from build123d import *

# Parameters (mm, degrees)
IZIM1_W                     = 40
IZIM1_H                     = 48
Y_KSEKLIK_EKSTR_ZYON1_DEPTH = 16
RADYUS4_R                   = 4
IZIM5_W                     = 24
IZIM5_H                     = 8
KES_EKSTR_ZYON1_DEPTH       = 59
IZIM6_W                     = 55
IZIM6_H                     = 32
Y_KSEKLIK_EKSTR_ZYON4_DEPTH = 12
RADYUS7_R                   = 10
IZIM9_R                     = 4.2
KES_EKSTR_ZYON2_DEPTH       = 21
IZIM10_W                    = 7
IZIM10_H                    = 35
Y_KSEKLIK_EKSTR_ZYON5_DEPTH = 16
KES_EKSTR_ZYON3_DEPTH       = 16


with BuildPart() as part:
    # Çizim1 → Yükseklik-Ekstrüzyon1 (new body)
    with BuildSketch(Plane.XY):
        with Locations((-20, 24)):
            Rectangle(IZIM1_W, IZIM1_H)
    extrude(amount=Y_KSEKLIK_EKSTR_ZYON1_DEPTH)

    # Radyus4
    radyus4_edges = [part.edges().sort_by_distance(p)[0] for p in [
        (-40, 24, 16),
        (0, 24, 16),
    ]]
    fillet(radyus4_edges, radius=RADYUS4_R)

    # Çizim5 → Kes-Ekstrüzyon1 (cut)
    with BuildSketch(Plane(origin=(0, 48, 0), x_dir=(1, 0, 0), z_dir=(0, 1, 0))):
        with Locations((-20, -4)):
            Rectangle(IZIM5_W, IZIM5_H)
    extrude(amount=-KES_EKSTR_ZYON1_DEPTH, mode=Mode.SUBTRACT)

    # Çizim6 → Yükseklik-Ekstrüzyon4 (add)
    with BuildSketch(Plane.XZ):
        with Locations((-20, 16)):
            Rectangle(IZIM6_W, IZIM6_H)
    extrude(amount=Y_KSEKLIK_EKSTR_ZYON4_DEPTH)

    # Radyus7
    radyus7_edges = [part.edges().sort_by_distance(p)[0] for p in [
        (7.5, -6, 32),
        (-47.5, -6, 32),
    ]]
    fillet(radyus7_edges, radius=RADYUS7_R)

    # Çizim9 → Kes-Ekstrüzyon2 (cut)
    with BuildSketch(Plane.XZ.offset(12)):
        with Locations((-37.5, 22)):
            Circle(IZIM9_R)
        with Locations((-2.5, 22)):
            Circle(IZIM9_R)
    extrude(amount=-KES_EKSTR_ZYON2_DEPTH, mode=Mode.SUBTRACT)

    # Çizim10 → Yükseklik-Ekstrüzyon5 (add)
    with BuildSketch(Plane.XY.offset(16)):
        with Locations((-19.227636849, 17.5)):
            Rectangle(IZIM10_W, IZIM10_H)
    extrude(amount=Y_KSEKLIK_EKSTR_ZYON5_DEPTH)

    # Çizim11 → Kes-Ekstrüzyon3 (cut)
    with BuildSketch(Plane(origin=(-15.727636849, 0, 0), x_dir=(0, 0, -1), z_dir=(1, 0, 0))):
        Polygon((-16, 35), (-32, 0), (-32, 35), align=None)
    extrude(amount=-KES_EKSTR_ZYON3_DEPTH, mode=Mode.SUBTRACT)


solid = part.part
Can you work these out from the model? Positions are in its coordinate system, mm. A direction names the side the tool comes from. Give positions to 0.01 mm unless a question says otherwise; leave off trailing zeros. Loops run counter-clockwise (first coordinate to the right, second up) from the corner with the lowest first, then second, coordinate; pieces in that order, holes last. Notation, with made-up numbers: (17.25, 16) - (33.25, 16) arc R21 cw to (33.25, 29) - close; hole circle Ø6 at (47, 9.5). An arc over 180 degrees is marked (long way). Return JSON: item names as keys, results as strings.
1. For faces 1 (the face through (-40, 24, 6)), 2 (the face through (-4.3, 0, 16.2)), 3 (the face through (-22.728, 13, 22)), 4 (the face through (-8, 24, 4)), 5 (the face through (-24, 24, 16)), which set-ups out of +Z, -Z, +X, -X, +Y, -Y let a thin tool reach every point of the face, with its end or its side?
Output values:
{"face 1": "+Z, -Z, -X, +Y", "face 2": "+Z, +X, +Y", "face 3": "+Z, -X, +Y", "face 4": "-Z, +Y", "face 5": "+Z, +Y"}
2. I want a section at A-A on z = 21. Please give me the cut outline in (x, y), and give its area (3 significant figures).
Output values:
{"outline": "(-47.5, -12) - (-41.58, -12) - (-41.58, 0) - (-47.5, 0) - close; (-33.42, -12) - (-6.58, -12) - (-6.58, 0) - (-15.73, 0) - (-15.73, 24.06) - (-22.73, 24.06) - (-22.73, 0) - (-33.42, 0) - close; (1.58, -12) - (7.5, -12) - (7.5, 0) - (1.58, 0) - close", "area": "633 mm²"}
3. I want a section at D-D on z = 14. Please give me the cut outline in (x, y).
Output values:
{"outline": "(-47.5, -12) - (7.5, -12) - (7.5, 0) - (-0.54, 0) - (-0.54, 48) - (-39.46, 48) - (-39.46, 0) - (-47.5, 0) - close"}
4. I want a section at B-B on x = -27. Please give me the cut outline in (y, z), and give its area (3 significant figures).
Output values:
{"outline": "(-12, 0) - (0, 0) - (0, 8) - (48, 8) - (48, 16) - (0, 16) - (0, 32) - (-12, 32) - close", "area": "768 mm²"}
5. I want a section at C-C on y = 40. Please give me the cut outline in (x, z).
Output values:
{"outline": "(-40, 0) - (-32, 0) - (-32, 8) - (-8, 8) - (-8, 0) - (0, 0) - (0, 12) arc R4 ccw to (-4, 16) - (-36, 16) arc R4 ccw to (-40, 12) - close"}
6. If I drill on line 1 (Z direction, x = -37.5, y = -7.75); line 2 (X direction, y = 2, z = 2.5); line 3 (Y direction, x = -45, z = 13), over which ranges is the centre line in solid material (lowest first)?
Output values:
{"line 1": "z = 0 to 17.8, 26.2 to 32", "line 2": "x = -40 to -32, -8 to 0", "line 3": "y = -12 to 0"}
7. We'd pull the mould along Z, two halves only. Please class faces 6 (the face through (-20, 0, 4)), 7 (the face through (-3.047, -6.084, 26.164)), 8 (the face through (-20, 24, 8)), 9 (the face through (-20, -6, 32)): +Z half, -Z half, draft (parallel to the pull), parting line (faces both ways), or undercut.
Output values:
{"face 6": "draft", "face 7": "undercut", "face 8": "-Z half", "face 9": "+Z half"}
8. I'm going to push flat-ended pins straight in: pin 1 Ø6.5 at (y, z) = (17.5, 5.5) entering from +X; pin 2 Ø10 at (y, z) = (19, 17.5) entering from -X; pin 3 Ø2.5 at (x, z) = (-22.5, 5.5) entering from +Y. Where does each tip first touch, or does it pass through?
Output values:
{"pin 1": "stops at x = 0", "pin 2": "stops at x = -39.97", "pin 3": "stops at y = 0"}
